Part model, mm, in its own coordinate system. Give positions to 0.01 mm unless a question says otherwise; leave off trailing zeros. Loops run counter-clockwise (first coordinate to the right, second up) from the corner with the lowest first, then second, coordinate; pieces in that order, holes last. Notation, with made-up numbers: M 81.5,23 L 90.5,23 A17 cw 90.5,46 Z; hole C 50,-24.75 d7. An arc over 180 degrees is marked long. Put each result on its own line as item: value. Start each with the question number.
```python
from build123d import *

# Parameters (mm, degrees)
SKETCH1_W           = 90
SKETCH1_H           = 22
SKETCH1_R           = 1.5
BOSS_EXTRUDE1_DEPTH = 1.5


with BuildPart() as part:
    # Sketch1 → Boss-Extrude1 (new body)
    with BuildSketch(Plane(origin=(0, 0, 0), x_dir=(1, 0, 0), z_dir=(0, 1, 0))):
        Rectangle(SKETCH1_W, SKETCH1_H)
        with Locations(Location((35.565, -1, 0), (0, 0, 270))):
            Circle(SKETCH1_R, mode=Mode.SUBTRACT)
        with Locations(Location((-35.565, -1, 0), (0, 0, 270))):
            Circle(SKETCH1_R, mode=Mode.SUBTRACT)
    extrude(amount=-BOSS_EXTRUDE1_DEPTH)


solid = part.part
```
1) Band-saw the part on A-A on z = 1. Give the cut face in (x, y) (3 decimals).
2) Mould opens along X. For faces 1 (the cylindrical face through (36.579, -0.74, -0.106)), 2 (the flat face through (-1, -1, -11)), 3 (the flat face through (-45, -1, 0)) say: +X half, -X half, draft (parallel to the pull), parting line (faces both ways), or undercut.
3) Wall check: L1, parallel to X at y = -1.1, z = 1 (3 decimals); L2, parallel to X at y = -0.1, z = 2; L3, parallel to Z at x = -34.5, y = -0.15. Give the ranges that are in metal, low to high.
Evaluation:
1. outline: M -45,-1.5 L -37.065,-1.5 L -37.065,0 L -45,0 Z; M -34.065,-1.5 L 34.065,-1.5 L 34.065,0 L -34.065,0 Z; M 37.065,-1.5 L 45,-1.5 L 45,0 L 37.065,0 Z
2. face 1: undercut
2. face 2: draft
2. face 3: -X half
3. L1: -45 to -37.065, -34.065 to 34.065, 37.065 to 45
3. L2: -45 to -36.68, -34.45 to 34.45, 36.68 to 45
3. L3: -11 to -0.06, 2.06 to 11
